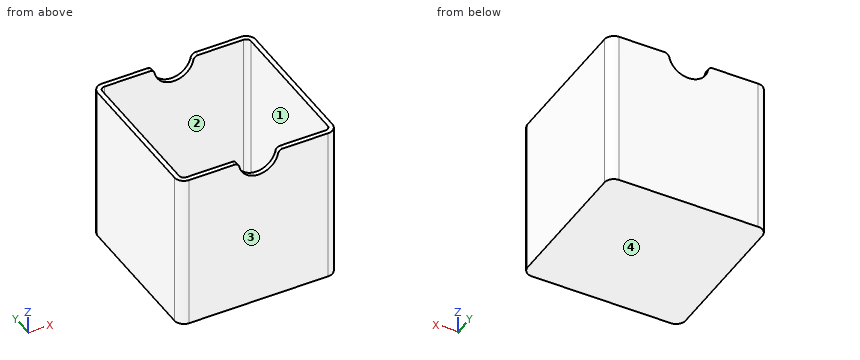
```python
from build123d import *

# Parameters (mm, degrees)
F0_W     = 100
F0_H     = 100
F1_DEPTH = 100
F2_R     = 6
F3_T     = -3
F4_R     = 12.5
F5_DEPTH = 100.001
F6_R     = 3


with BuildPart() as f1:
    # F0 (on Top) → F1 (new body)
    with BuildSketch(Plane.XY):
        Rectangle(F0_W, F0_H)
    extrude(amount=F1_DEPTH)

    # F2
    f2_edges = [f1.edges().sort_by_distance(p)[0] for p in [
        (50, -50, 50),
        (-50, -50, 50),
        (50, 50, 50),
        (-50, 50, 50),
    ]]
    fillet(f2_edges, radius=F2_R)

    # F3
    f3_openings = [f1.faces().sort_by_distance(p)[0] for p in [
        (0, 0, 100),
    ]]
    offset(amount=F3_T, openings=f3_openings)

    # F4 (on face) → F5 (cut, through all)
    with BuildSketch(Plane.XZ.offset(50)):
        with Locations((0, 100)):
            Circle(F4_R)
    extrude(amount=-F5_DEPTH, mode=Mode.SUBTRACT)

    # F6
    f6_edges = [f1.edges().sort_by_distance(p)[0] for p in [
        (-12.5, 48.5, 100),
        (-12.5, -48.5, 100),
        (12.5, -48.5, 100),
        (12.5, 48.5, 100),
    ]]
    fillet(f6_edges, radius=F6_R)


solid = f1.part
```
Part model, mm, in its own coordinate system. Face numbers are marked on the shaded views. Give positions to 0.01 mm unless a question says otherwise; leave off trailing zeros. Loops run counter-clockwise (first coordinate to the right, second up) from the corner with the lowest first, then second, coordinate; pieces in that order, holes last. Notation, with made-up numbers: M -23.75,45 L 18.25,45 A22 ccw 18.25,80 Z; hole C 67,-31.75 d9. An arc over 180 degrees is marked long. Return JSON: item names as keys, results as strings.
1) Pull direction Y, two halves, no side cores. Call the marked faces 1, 2, 3 and 4: released by +Y, released by -Y, zero draft, split by the parting line, or undercut.
Calculated:
{"face 1": "undercut", "face 2": "undercut", "face 3": "released by -Y", "face 4": "zero draft"}
2) Flat gauge pin, fed straight in: pin 1 Ø10 at (x, y) = (-19, 14.5) entering from +Z. Where does the tip first touch, or does it go through?
Calculated:
{"pin 1": "stops at z = 3"}
3) Saw through at B-B, the plane z = 62.5. List the corners of the cut face in (x, y).
Calculated:
{"outline": "M -50,-44 A6 ccw -44,-50 L 44,-50 A6 ccw 50,-44 L 50,44 A6 ccw 44,50 L -44,50 A6 ccw -50,44 Z; hole M -47,-44 A3 ccw -44,-47 L 44,-47 A3 ccw 47,-44 L 47,44 A3 ccw 44,47 L -44,47 A3 ccw -47,44 Z"}
4) Saw through at D-D, the plane z = 89.5. List the corners of the cut face in (x, y).
Calculated:
{"outline": "M -50,-44 A6 ccw -44,-50 L -6.78,-50 L -6.78,-47 L -44,-47 A3 cw -47,-44 L -47,44 A3 cw -44,47 L -6.78,47 L -6.78,50 L -44,50 A6 ccw -50,44 Z; M 6.78,-50 L 44,-50 A6 ccw 50,-44 L 50,44 A6 ccw 44,50 L 6.78,50 L 6.78,47 L 44,47 A3 cw 47,44 L 47,-44 A3 cw 44,-47 L 6.78,-47 Z"}
5) Saw through at C-C, the plane y = 40. List the corners of the cut face in (x, z), then the cut area to 3 significant figures.
Calculated:
{"outline": "M -50,0 L 50,0 L 50,100 L 47,100 L 47,3 L -47,3 L -47,100 L -50,100 Z", "area": "882 mm2"}
6) Saw through at A-A, the plane x = 3.5. List the corners of the cut face in (y, z).
Calculated:
{"outline": "M -50,0 L 50,0 L 50,88 L 47,88 L 47,3 L -47,3 L -47,88 L -50,88 Z"}
7) Drill centre lines: line 1 (X direction, y = -43, z = 42); line 2 (Z direction, x = 15, y = 32). Where is each one in solid material? Low to high.
Calculated:
{"line 1": "x = -50 to -47, 47 to 50", "line 2": "z = 0 to 3"}
